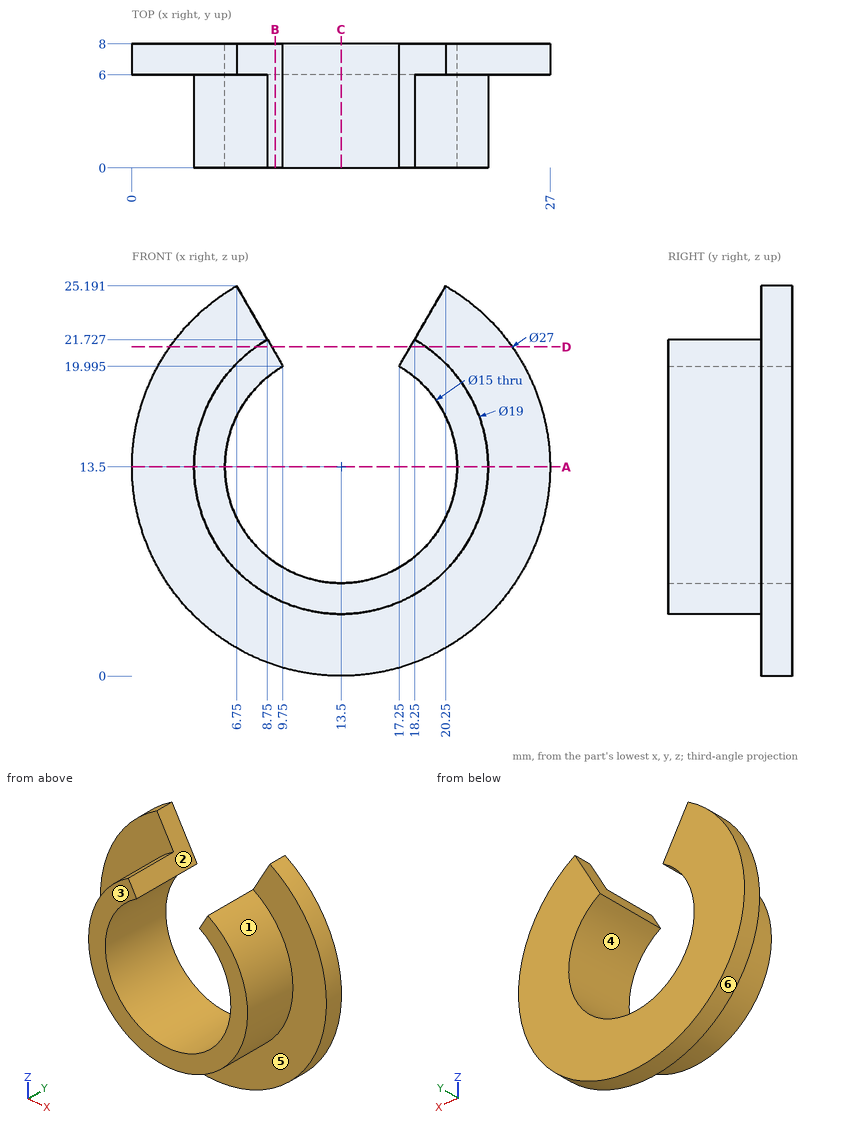
Job drawing, mm, ordinate dimensions from the low corner. One solid piece. A direction names the side the tool comes from. Round coordinates to 2 decimals unless told otherwise and drop trailing zeros. Write each loop counter-clockwise with the first axis right and the second up, starting at its lowest first coordinate (ties: lowest second). Pieces come first, ordered by that corner, then holes. Notation, with made-up numbers: M -37.5,51 L 10.5,51 A21 ccw 10.5,72 Z; hole C 47.5,-30 d3. An arc over 180 degrees is marked long. Return JSON: item names as keys, results as strings. Group by question number.
(1) Saw through at A-A on z = 13.5. Write the cut outline in (x, y).
(2) Pin check, flat tips, straight feed: pin 1 Ø3 at (y, z) = (2.5, 9) entering from +X; pin 2 Ø1.5 at (y, z) = (5.5, 16.5) entering from -X. Stop position of each tip, or through.
(3) Saw through at B-B on x = 9.25. Write the cut outline in (y, z).
(4) Two-plate mould, pull along Z, no slides. Class the marked faces 4, 5 and 6: +Z half, -Z half, draft (parallel to the pull), parting line (faces both ways), or undercut.
(5) Saw through at C-C on x = 13.5. Write the cut outline in (y, z).
(6) Which spindle directions (+Z, -Z, +X, -X, +Y, -Y) get a long thin tool onto all of the face, cutting with end or side? Do the marked faces 1, 2 and 3. Say none if no direction does.
(7) Saw through at D-D on z = 21.25. Write the cut outline in (x, y) (1 decimal).
(8) Drill centre lines: probe 1 along Z at (x, y) = (13.25, 4.75); probe 2 along X at (y, z) = (4.75, 9.25) (1 decimal); probe 3 along X at (y, z) = (7.25, 18.5). Where is each one in solid material? Low to high.
Returned:
{
 "1": {"outline": "M 0,6 L 4,6 L 4,0 L 6,0 L 6,8 L 0,8 Z; M 21,0 L 23,0 L 23,6 L 27,6 L 27,8 L 21,8 Z"},
 "2": {"pin 1": "x = 22.51", "pin 2": "x = 0.22"},
 "3": {"outline": "M 0,5 L 6,5 L 6,0.69 L 8,0.69 L 8,7.32 L 0,7.32 Z; M 0,19.68 L 8,19.68 L 8,20.86 L 0,20.86 Z"},
 "4": {"face 4": "undercut", "face 5": "draft", "face 6": "parting line"},
 "5": {"outline": "M 0,4 L 6,4 L 6,0 L 8,0 L 8,6 L 0,6 Z"},
 "6": {"face 1": "-Y", "face 2": "+Z, +Y, -Y", "face 3": "+Z, -Z, +X, -X, -Y"},
 "7": {"outline": "M 2.4,6 L 8,6 L 8,0 L 9,0 L 9,8 L 2.4,8 Z; M 18,0 L 19,0 L 19,6 L 24.6,6 L 24.6,8 L 18,8 Z"},
 "8": {"probe 1": "4 to 6", "probe 2": "5 to 7.3, 19.7 to 22", "probe 3": "0.96 to 7.91, 19.09 to 26.04"}
}
